Here's how the part is built. I have some questions about the finished solid (model axes, mm). Coordinates: 2 decimals unless noted, no trailing zeros. Write each loop counter-clockwise with the first axis right and the second up, starting at its lowest first coordinate (ties: lowest second). Pieces come first, ordered by that corner, then holes.
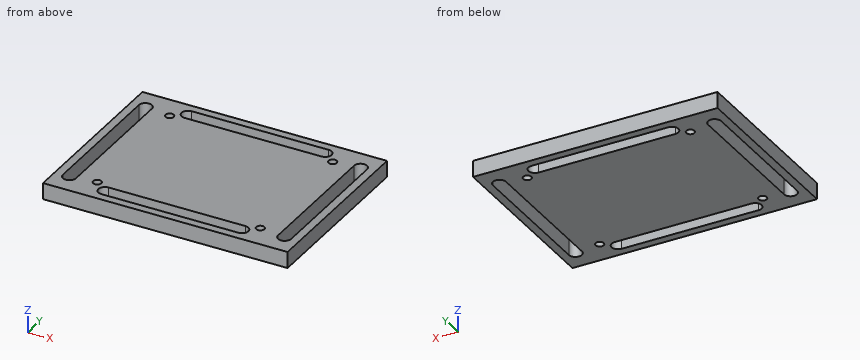
```python
from build123d import *

# Parameters (mm, degrees)
SKETCH1_W           = 75
SKETCH1_H           = 55
SKETCH1_R           = 1.25
BOSS_EXTRUDE1_DEPTH = 5


with BuildPart() as part:
    # Sketch1 → Boss-Extrude1 (new body)
    with BuildSketch(Plane.XY):
        Rectangle(SKETCH1_W, SKETCH1_H)
        with Locations((-25, 20)):
            Circle(SKETCH1_R, mode=Mode.SUBTRACT)
        with Locations((25, 20)):
            Circle(SKETCH1_R, mode=Mode.SUBTRACT)
        with Locations((25, -20)):
            Circle(SKETCH1_R, mode=Mode.SUBTRACT)
        with Locations((-25, -20)):
            Circle(SKETCH1_R, mode=Mode.SUBTRACT)
        with BuildLine():
            Line((-21, 25), (21, 25))
            ThreePointArc((21, 25), (23, 23), (21, 21))
            Line((21, 21), (-21, 21))
            ThreePointArc((-21, 21), (-23, 23), (-21, 25))
        make_face(mode=Mode.SUBTRACT)
        with BuildLine():
            Line((-21, -25), (21, -25))
            ThreePointArc((21, -25), (23, -23), (21, -21))
            Line((21, -21), (-21, -21))
            ThreePointArc((-21, -21), (-23, -23), (-21, -25))
        make_face(mode=Mode.SUBTRACT)
        with BuildLine():
            Line((-31, 21), (-31, -21))
            ThreePointArc((-31, -21), (-33, -23), (-35, -21))
            Line((-35, -21), (-35, 21))
            ThreePointArc((-35, 21), (-33, 23), (-31, 21))
        make_face(mode=Mode.SUBTRACT)
        with BuildLine():
            Line((31, 21), (31, -21))
            ThreePointArc((31, -21), (33, -23), (35, -21))
            Line((35, -21), (35, 21))
            ThreePointArc((35, 21), (33, 23), (31, 21))
        make_face(mode=Mode.SUBTRACT)
    extrude(amount=BOSS_EXTRUDE1_DEPTH)


solid = part.part
```
1) Imagine slicing it at D-D on y = 20. Please give me the cut outline in (x, z), then the cut area to 3 significant figures.
Values follow:
outline: (-37.5, 0) - (-35, 0) - (-35, 5) - (-37.5, 5) - close; (-31, 0) - (-26.25, 0) - (-26.25, 5) - (-31, 5) - close; (-23.75, 0) - (23.75, 0) - (23.75, 5) - (-23.75, 5) - close; (26.25, 0) - (31, 0) - (31, 5) - (26.25, 5) - close; (35, 0) - (37.5, 0) - (37.5, 5) - (35, 5) - close
area: 310 mm2
2) I need wall thicknesses on probe 1 along Y at (x, z) = (-5.5, 3.35); probe 2 along Y at (x, z) = (25, 3.3); probe 3 along X at (y, z) = (-7, 4.1). Which ranges of each line are inside material? Lowest first, please.
Values follow:
probe 1: y = -27.5 to -25, -21 to 21, 25 to 27.5
probe 2: y = -27.5 to -21.25, -18.75 to 18.75, 21.25 to 27.5
probe 3: x = -37.5 to -35, -31 to 31, 35 to 37.5
3) Imagine slicing it at C-C on z = 1.7. Count the separate pieces of the cut face and the enclosed holes in it, then the cut area to 3 significant figures.
Values follow:
separate pieces: 1
enclosed holes: 8
area: 3,380 mm2
4) Imagine slicing it at B-B on x = 25. Please give me the cut outline in (y, z).
Values follow:
outline: (-27.5, 0) - (-21.25, 0) - (-21.25, 5) - (-27.5, 5) - close; (-18.75, 0) - (18.75, 0) - (18.75, 5) - (-18.75, 5) - close; (21.25, 0) - (27.5, 0) - (27.5, 5) - (21.25, 5) - close
5) Will this pin go through, and if not, where does the flat tip stop? pin 1 (2 mm diameter, centred on x = 25, y = -20, fed in from -Z).
Values follow:
pin 1: passes through
6) Imagine slicing it at A-A on y = -17. Please give me the cut outline in (x, z), then the cut area to 3 significant figures.
Values follow:
outline: (-37.5, 0) - (-35, 0) - (-35, 5) - (-37.5, 5) - close; (-31, 0) - (31, 0) - (31, 5) - (-31, 5) - close; (35, 0) - (37.5, 0) - (37.5, 5) - (35, 5) - close
area: 335 mm2
